Print and shaded views of the part. All mm, measured from the part's lowest x, y and z. Coordinates: 2 decimals unless noted, no trailing zeros. Order: outer loops, then holes, each group sorted by start corner. A loop starts at its lowest first (then second) coordinate and runs counter-clockwise, first axis right, second up. Notation, with made-up numbers: (-17, 45.5) -> (16, 45.5) arc R15 cw to (16, 65.5) -> close; hole circle Ø5 at (55, 42.5). An arc over 180 degrees is marked (long way). Return JSON: item names as keys, results as strings. Group by question number.
1) Flat gauge pin, fed straight in: pin 1 (3 mm diameter, centred on x = 11.5, y = 13, fed in from -Z). Where does the tip first touch, or does it go through?
2) Cut at D-D (x = 7.5). Write the cut outline in (y, z), and give its area (3 significant figures).
3) Cut at B-B (y = 6). Write the cut outline in (x, z).
4) Cut at A-A (x = 27.25). Write the cut outline in (y, z), and give its area (3 significant figures).
5) Probe line 1 (X direction, y = 10, z = 2.05); line 2 (Y direction, x = 27.25, z = 1.05); line 3 (Y direction, x = 3.5, z = 2.25). List the from-to ranges inside material, lowest first.
6) Cut at C-C (z = 0.9). Write the cut outline in (x, y), and give its area (3 significant figures).
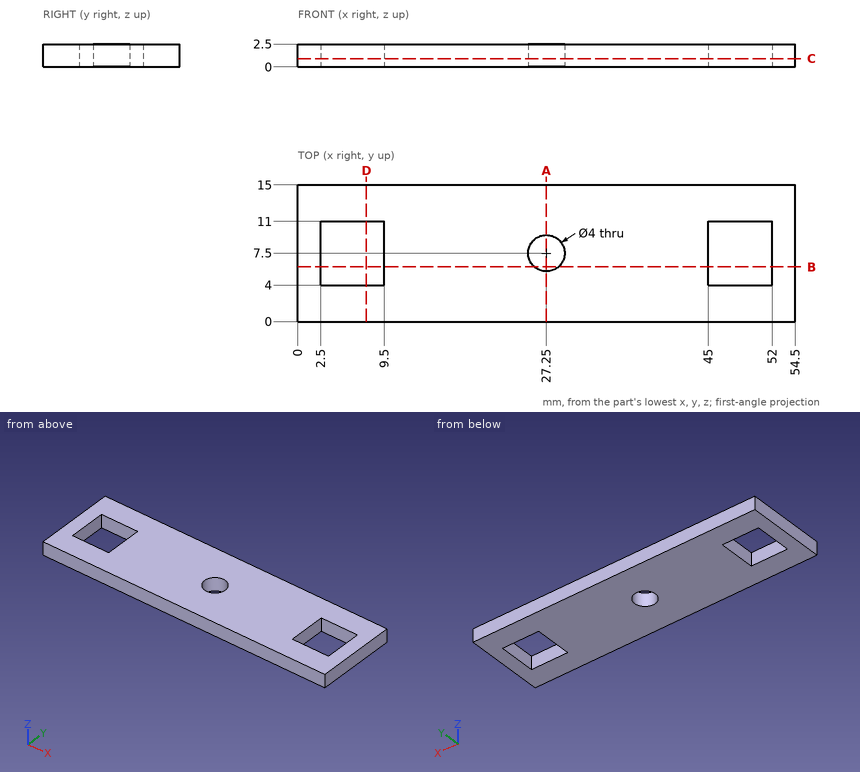
Answers below:
{
 "1": {"pin 1": "stops at z = 0"},
 "2": {"outline": "(0, 0) -> (4, 0) -> (4, 2.5) -> (0, 2.5) -> close; (11, 0) -> (15, 0) -> (15, 2.5) -> (11, 2.5) -> close", "area": "20.0 mm^2"},
 "3": {"outline": "(0, 0) -> (2.5, 0) -> (2.5, 2.5) -> (0, 2.5) -> close; (9.5, 0) -> (25.93, 0) -> (25.93, 2.5) -> (9.5, 2.5) -> close; (28.57, 0) -> (45, 0) -> (45, 2.5) -> (28.57, 2.5) -> close; (52, 0) -> (54.5, 0) -> (54.5, 2.5) -> (52, 2.5) -> close"},
 "4": {"outline": "(0, 0) -> (5.5, 0) -> (5.5, 2.5) -> (0, 2.5) -> close; (9.5, 0) -> (15, 0) -> (15, 2.5) -> (9.5, 2.5) -> close", "area": "27.5 mm^2"},
 "5": {"line 1": "x = 0 to 2.5, 9.5 to 45, 52 to 54.5", "line 2": "y = 0 to 5.5, 9.5 to 15", "line 3": "y = 0 to 4, 11 to 15"},
 "6": {"outline": "(0, 0) -> (54.5, 0) -> (54.5, 15) -> (0, 15) -> close; hole (2.5, 4) -> (9.5, 4) -> (9.5, 11) -> (2.5, 11) -> close; hole circle Ø4 at (27.25, 7.5); hole (45, 4) -> (52, 4) -> (52, 11) -> (45, 11) -> close", "area": "707 mm^2"}
}
